```python
from build123d import *

# Parameters (mm, degrees)
F0_W     = 200
F0_H     = 3.1
F1_DEPTH = 3


with BuildPart() as f1:
    # F0 (on Top) → F1 (new body)
    with BuildSketch(Plane.XY):
        Polygon((7.45, -20), (116, -20), (116, -7.45), (112.95, -7.45), (112.95, 7.45), (116, 7.45), (116, 20), (7.45, 20), (7.45, 16.95), (-7.45, 16.95), (-7.45, 20), (-116, 20), (-116, 7.45), (-112.95, 7.45), (-112.95, -7.45), (-116, -7.45), (-116, -20), (-7.45, -20), (-7.45, -16.95), (7.45, -16.95), align=None)
        Rectangle(F0_W, F0_H, mode=Mode.SUBTRACT)
    extrude(amount=F1_DEPTH)


solid = f1.part
```
Geometry: final body of the model. Coordinates: model frame, mm. Round coordinates to 2 decimals unless told otherwise and drop trailing zeros. Write each loop counter-clockwise with the first axis right and the second up, starting at its lowest first coordinate (ties: lowest second). Pieces come first, ordered by that corner, then holes.
Item 1: Material intervals for L1, parallel to X at y = 17, z = 1.5; L2, parallel to Y at x = 82.5, z = 1.7; L3, parallel to Y at x = -1, z = 1.5, sorted ascending.
Item 2: Section query B-B (z = 0.45). Return loops of the section in (x, y).
Item 3: Section query A-A (x = -94). Return loops of the section in (y, z), plus the area to 3 significant figures.
Item 4: Pin query (flat end, axial travel): P1, Ø1.5, axis at x = -2.5, z = 2, coming from the -Y side; P2, Ø1.5, axis at y = -3, z = 1, coming from the +X side; P3, Ø1.5, axis at y = 0.5, z = 2, coming from the -X side. Return the tip coordinate at first contact, or that it passes through.
Completed:
1. L1: x = -116 to -7.45, 7.45 to 116
1. L2: y = -20 to -1.55, 1.55 to 20
1. L3: y = -16.95 to -1.55, 1.55 to 16.95
2. outline: (-116, -20) - (-7.45, -20) - (-7.45, -16.95) - (7.45, -16.95) - (7.45, -20) - (116, -20) - (116, -7.45) - (112.95, -7.45) - (112.95, 7.45) - (116, 7.45) - (116, 20) - (7.45, 20) - (7.45, 16.95) - (-7.45, 16.95) - (-7.45, 20) - (-116, 20) - (-116, 7.45) - (-112.95, 7.45) - (-112.95, -7.45) - (-116, -7.45) - close; hole (-100, -1.55) - (100, -1.55) - (100, 1.55) - (-100, 1.55) - close
3. outline: (-20, 0) - (-1.55, 0) - (-1.55, 3) - (-20, 3) - close; (1.55, 0) - (20, 0) - (20, 3) - (1.55, 3) - close
3. area: 111 mm2
4. P1: stops at y = -16.95
4. P2: stops at x = 112.95
4. P3: stops at x = -112.95
